Read the model definition and answer for the solid it produces. Units are mm, in the model's axes. Face numbers are marked on the shaded views. Round coordinates to 2 decimals unless told otherwise and drop trailing zeros. Order: outer loops, then holes, each group sorted by start corner. A loop starts at its lowest first (then second) coordinate and runs counter-clockwise, first axis right, second up. Notation, with made-up numbers: (9.25, 43.5) -> (26.25, 43.5) arc R14 ccw to (26.25, 57.5) -> close; hole circle Ø2 at (-8, 89). An arc over 180 degrees is marked (long way). One line per item, written item: value. Start each with the question number.
1. Consider line 1 (Y direction, x = -48, z = 13.5); line 2 (Y direction, x = -37, z = 13.25); line 3 (Y direction, x = -83.3, z = 5.75). Determine where each line is inside the solid, lowest interval first.
2. Section A-A (x = -89.25) is taken. Give the vertices of the cut face in (y, z), then the cut area to 3 significant figures.
3. Flat-ended cylindrical pins translate along their axes: pin 1 Ø14.5 at (x, y) = (-77.35, -10.31) entering from +Z; pin 2 Ø6 at (x, z) = (-91, 5.5) entering from -Y; pin 3 Ø1 at (y, z) = (-72.5, 5.5) entering from +X; pin 4 Ø1 at (x, y) = (-58, -32.5) entering from +Z. Find the tip coordinate at first contact, or state that the pin passes through.
4. Section B-B (y = -29) is taken. State how many separate pieces and enclosed holes the cut face has, then the cut area to 3 significant figures.
5. The mould has two halves that part along Y. Classify the marked faces 1 and 2: released by +Y, released by -Y, zero draft, split by the parting line, or undercut.
6. Section C-C (y = -64) is taken. Give the vertices of the cut face in (x, z).
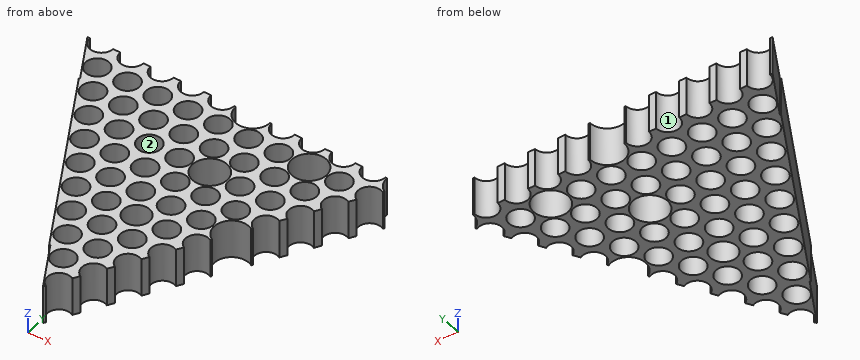
from build123d import *

# Parameters (mm, degrees)
F0_R     = 4.55
F0_R_2   = 5.099371
F0_R_3   = 6.75
F1_DEPTH = 15


with BuildPart() as f1:
    # F0 (on Top) → F1 (new body)
    with BuildSketch(Plane.XY):
        with BuildLine():
            Line((-114.5, -18.186533), (-73, -90.066642))
            Line((-73, -90.066642), (-72.65359, -89.866642))
            Line((-72.65359, -89.866642), (-62.26906, -107.853175))
            Line((-62.26906, -107.853175), (-61.775, -106.997439))
            ThreePointArc((-61.775, -106.997439), (-63.440416, -100.782023), (-57.225, -99.116607))
            Line((-57.225, -99.116607), (-55.825, -96.691736))
            ThreePointArc((-55.825, -96.691736), (-57.490416, -90.476321), (-51.275, -88.810905))
            Line((-51.275, -88.810905), (-49.875, -86.386034))
            ThreePointArc((-49.875, -86.386034), (-51.540416, -80.170618), (-45.325, -78.505203))
            Line((-45.325, -78.505203), (-43.925, -76.080332))
            ThreePointArc((-43.925, -76.080332), (-45.590416, -69.864916), (-39.375, -68.199501))
            Line((-39.375, -68.199501), (-37.975, -65.774629))
            ThreePointArc((-37.975, -65.774629), (-39.640416, -59.559214), (-33.425, -57.893798))
            Line((-33.425, -57.893798), (-33.125, -57.374183))
            ThreePointArc((-33.125, -57.374183), (-35.595671, -48.153512), (-26.375, -45.68284))
            Line((-26.375, -45.68284), (-26.075, -45.163225))
            ThreePointArc((-26.075, -45.163225), (-27.740416, -38.947809), (-21.525, -37.282394))
            Line((-21.525, -37.282394), (-20.125, -34.857523))
            ThreePointArc((-20.125, -34.857523), (-21.790416, -28.642107), (-15.575, -26.976691))
            Line((-15.575, -26.976691), (-14.175, -24.55182))
            ThreePointArc((-14.175, -24.55182), (-15.840416, -18.336405), (-9.625, -16.670989))
            Line((-9.625, -16.670989), (-8.225, -14.246118))
            ThreePointArc((-8.225, -14.246118), (-9.890416, -8.030702), (-3.675, -6.365287))
            Line((-3.675, -6.365287), (-3.375, -5.845671))
            ThreePointArc((-3.375, -5.845671), (-5.845671, -3.375), (-6.75, 0))
            Line((-6.75, 0), (-7.35, 0))
            ThreePointArc((-7.35, 0), (-11.9, -4.55), (-16.45, 0))
            Line((-16.45, 0), (-19.25, 0))
            ThreePointArc((-19.25, 0), (-23.8, -4.55), (-28.35, 0))
            Line((-28.35, 0), (-31.15, 0))
            ThreePointArc((-31.15, 0), (-35.7, -4.55), (-40.25, 0))
            Line((-40.25, 0), (-43.05, 0))
            ThreePointArc((-43.05, 0), (-47.6, -4.55), (-52.15, 0))
            Line((-52.15, 0), (-52.75, 0))
            ThreePointArc((-52.75, 0), (-59.5, -6.75), (-66.25, 0))
            Line((-66.25, 0), (-66.85, 0))
            ThreePointArc((-66.85, 0), (-71.4, -4.55), (-75.95, 0))
            Line((-75.95, 0), (-78.75, 0))
            ThreePointArc((-78.75, 0), (-83.3, -4.55), (-87.85, 0))
            Line((-87.85, 0), (-90.65, 0))
            ThreePointArc((-90.65, 0), (-95.2, -4.55), (-99.75, 0))
            Line((-99.75, 0), (-102.55, 0))
            ThreePointArc((-102.55, 0), (-107.1, -4.55), (-111.65, 0))
            Line((-111.65, 0), (-114.45, 0))
            ThreePointArc((-114.45, 0), (-119, -4.55), (-123.55, 0))
            Line((-123.55, 0), (-124.53812, 0))
            Line((-124.53812, 0), (-114.15359, -17.986533))
            Line((-114.15359, -17.986533), (-114.5, -18.186533))
        make_face()
        with Locations((-65.45, -92.751321)):
            Circle(F0_R, mode=Mode.SUBTRACT)
        with Locations((-71.4, -82.445618)):
            Circle(F0_R, mode=Mode.SUBTRACT)
        with Locations((-59.5, -82.445618)):
            Circle(F0_R, mode=Mode.SUBTRACT)
        with Locations((-77.35, -72.139916)):
            Circle(F0_R, mode=Mode.SUBTRACT)
        with Locations((-65.45, -72.139916)):
            Circle(F0_R, mode=Mode.SUBTRACT)
        with Locations((-83.3, -61.834214)):
            Circle(F0_R, mode=Mode.SUBTRACT)
        with Locations((-89.25, -51.528512)):
            Circle(F0_R, mode=Mode.SUBTRACT)
        with Locations((-77.35, -51.528512)):
            Circle(F0_R, mode=Mode.SUBTRACT)
        with Locations((-71.4, -61.834214)):
            Circle(F0_R, mode=Mode.SUBTRACT)
        with Locations((-59.5, -61.834214)):
            Circle(F0_R_2, mode=Mode.SUBTRACT)
        with Locations((-65.45, -51.528512)):
            Circle(F0_R, mode=Mode.SUBTRACT)
        with Locations((-53.55, -72.139916)):
            Circle(F0_R, mode=Mode.SUBTRACT)
        with Locations((-47.6, -61.834214)):
            Circle(F0_R, mode=Mode.SUBTRACT)
        with Locations((-53.55, -51.528512)):
            Circle(F0_R, mode=Mode.SUBTRACT)
        with Locations((-41.65, -51.528512)):
            Circle(F0_R, mode=Mode.SUBTRACT)
        with Locations((-95.2, -41.222809)):
            Circle(F0_R, mode=Mode.SUBTRACT)
        with Locations((-101.15, -30.917107)):
            Circle(F0_R, mode=Mode.SUBTRACT)
        with Locations((-83.3, -41.222809)):
            Circle(F0_R, mode=Mode.SUBTRACT)
        with Locations((-71.4, -41.222809)):
            Circle(F0_R, mode=Mode.SUBTRACT)
        with Locations((-59.5, -41.222809)):
            Circle(F0_R, mode=Mode.SUBTRACT)
        with Locations((-89.25, -30.917107)):
            Circle(F0_R, mode=Mode.SUBTRACT)
        with Locations((-77.35, -30.917107)):
            Circle(F0_R, mode=Mode.SUBTRACT)
        with Locations((-65.45, -30.917107)):
            Circle(F0_R, mode=Mode.SUBTRACT)
        with Locations((-113.05, -10.305702)):
            Circle(F0_R, mode=Mode.SUBTRACT)
        with Locations((-107.1, -20.611405)):
            Circle(F0_R, mode=Mode.SUBTRACT)
        with Locations((-95.2, -20.611405)):
            Circle(F0_R, mode=Mode.SUBTRACT)
        with Locations((-101.15, -10.305702)):
            Circle(F0_R, mode=Mode.SUBTRACT)
        with Locations((-83.3, -20.611405)):
            Circle(F0_R, mode=Mode.SUBTRACT)
        with Locations((-89.25, -10.305702)):
            Circle(F0_R, mode=Mode.SUBTRACT)
        with Locations((-77.35, -10.305702)):
            Circle(F0_R, mode=Mode.SUBTRACT)
        with Locations((-71.4, -20.611405)):
            Circle(F0_R, mode=Mode.SUBTRACT)
        with Locations((-59.5, -20.611405)):
            Circle(F0_R, mode=Mode.SUBTRACT)
        with Locations((-65.45, -10.305702)):
            Circle(F0_R, mode=Mode.SUBTRACT)
        with Locations((-47.6, -41.222809)):
            Circle(F0_R, mode=Mode.SUBTRACT)
        with Locations((-35.7, -41.222809)):
            Circle(F0_R, mode=Mode.SUBTRACT)
        with Locations((-53.55, -30.917107)):
            Circle(F0_R_3, mode=Mode.SUBTRACT)
        with Locations((-41.65, -30.917107)):
            Circle(F0_R, mode=Mode.SUBTRACT)
        with Locations((-29.75, -30.917107)):
            Circle(F0_R, mode=Mode.SUBTRACT)
        with Locations((-47.6, -20.611405)):
            Circle(F0_R, mode=Mode.SUBTRACT)
        with Locations((-53.55, -10.305702)):
            Circle(F0_R, mode=Mode.SUBTRACT)
        with Locations((-35.7, -20.611405)):
            Circle(F0_R, mode=Mode.SUBTRACT)
        with Locations((-41.65, -10.305702)):
            Circle(F0_R, mode=Mode.SUBTRACT)
        with Locations((-29.75, -10.305702)):
            Circle(F0_R_3, mode=Mode.SUBTRACT)
        with Locations((-23.8, -20.611405)):
            Circle(F0_R, mode=Mode.SUBTRACT)
        with Locations((-17.85, -10.305702)):
            Circle(F0_R, mode=Mode.SUBTRACT)
    extrude(amount=F1_DEPTH)


solid = f1.part
Answer:
1. line 1: -77.91 to -66.37, -57.3 to -45.76, -36.69 to -34.76, -27.08 to -25.14, -16.08 to -4.53
1. line 2: -57.47 to -45.58, -36.86 to -24.97, -16.25 to -4.36
1. line 3: -72.23 to -66.38, -57.28 to -45.77, -36.67 to -25.16, -16.06 to -4.55
2. outline: (-61.92, 0) -> (-56.08, 0) -> (-56.08, 15) -> (-61.92, 15) -> close; (-46.98, 0) -> (-35.47, 0) -> (-35.47, 15) -> (-46.98, 15) -> close; (-26.37, 0) -> (-14.86, 0) -> (-14.86, 15) -> (-26.37, 15) -> close; (-5.76, 0) -> (0, 0) -> (0, 15) -> (-5.76, 15) -> close
2. area: 519 mm^2
3. pin 1: z = 15
3. pin 2: y = -64.09
3. pin 3: x = -46.12
3. pin 4: through
4. separate pieces: 8
4. enclosed holes: 0
4. area: 357 mm^2
5. face 1: released by +Y
5. face 2: undercut
6. outline: (-88.05, 0) -> (-87.3, 0) -> (-87.3, 15) -> (-88.05, 15) -> close; (-79.3, 0) -> (-75.4, 0) -> (-75.4, 15) -> (-79.3, 15) -> close; (-67.4, 0) -> (-64.12, 0) -> (-64.12, 15) -> (-67.4, 15) -> close; (-54.88, 0) -> (-51.6, 0) -> (-51.6, 15) -> (-54.88, 15) -> close; (-43.6, 0) -> (-39.7, 0) -> (-39.7, 15) -> (-43.6, 15) -> close
